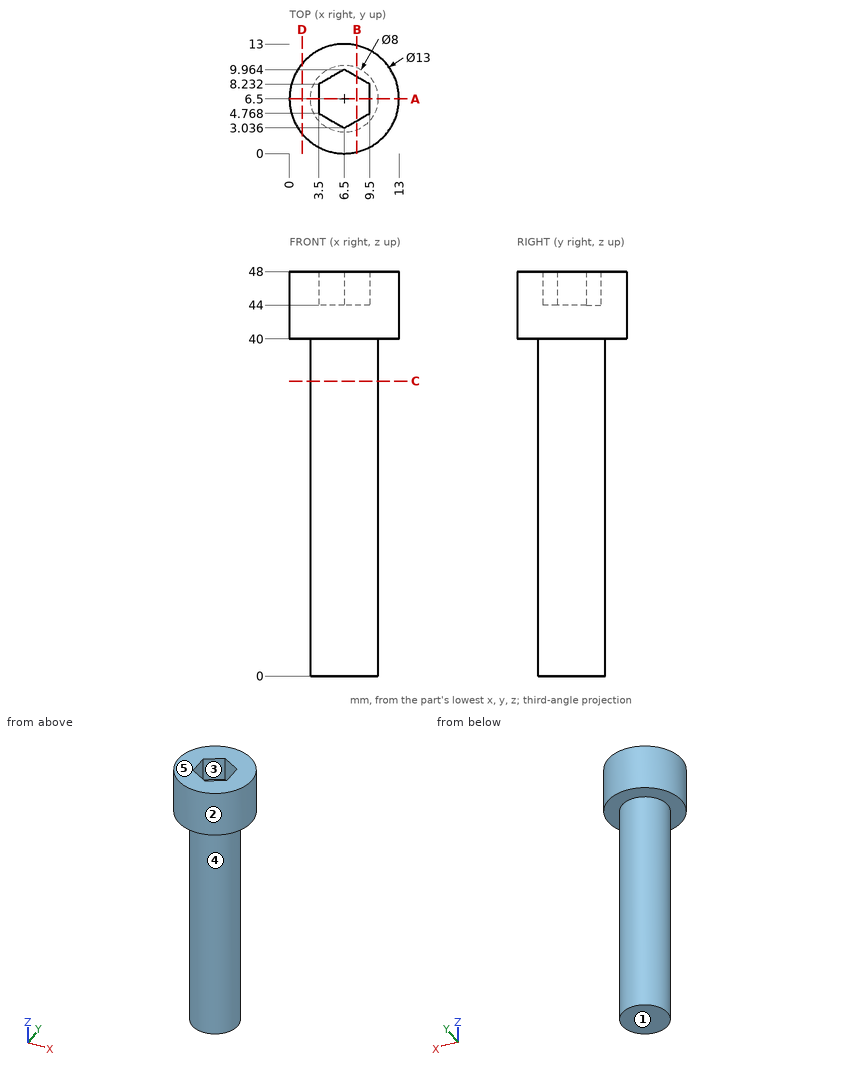
Source: three-view drawing plus pictorial views. Frame: mm from the lowest corner of the part. A direction names the side the tool comes from. Coordinates: 2 decimals unless noted, no trailing zeros. Order: outer loops, then holes, each group sorted by start corner. A loop starts at its lowest first (then second) coordinate and runs counter-clockwise, first axis right, second up. Notation, with made-up numbers: M 7.5,23.25 L 56.5,23.25 A28 cw 56.5,43.25 Z; hole C 1,-16.75 d9. An arc over 180 degrees is marked long. Answer in a Markdown table with one row per item.
(1) Material intervals for line 1 (Z direction, x = 6.5, y = 5); line 2 (Z direction, x = 12, y = 7); line 3 (Y direction, x = 6.25, z = 34), sorted ascending. Write a range as [from, to].
Numbers:
| item | result |
|---|---|
| line 1 | z = [0, 44] |
| line 2 | z = [40, 48] |
| line 3 | y = [2.51, 10.49] |
(2) Section query D-D, the plane x = 1.5. Output: boundary loops of the cut face in (y, z).
Numbers:
| item | result |
|---|---|
| outline | M 2.35,40 L 10.65,40 L 10.65,48 L 2.35,48 Z |
(3) Draft query along Y for the marked faces 1, 2 and 3. Return one class per face: pulls with the +Y half, pulls with the -Y half, needs draft (parallel to the pull), parting line crosses it, or undercut.
Numbers:
| item | result |
|---|---|
| face 1 | needs draft |
| face 2 | parting line crosses it |
| face 3 | undercut |
(4) Access query for the marked faces 4 and 5. Directions: +Z, -Z, +X, -X, +Y, -Y. A direction counts if a zero-diameter tool reaches every point of the face in a straight line with its end or side. Return the directions, or none.
Numbers:
| item | result |
|---|---|
| face 4 | -Z |
| face 5 | +Z, +X, -X, +Y, -Y |
(5) Section query C-C, the plane z = 35. Output: boundary loops of the cut face in (x, y).
Numbers:
| item | result |
|---|---|
| outline | C 6.5,6.5 d8 |
(6) Contact query for flat-ended pins moving along their axis: pin 1 Ø1.5 at (x, y) = (10.5, 6.5) entering from -Z; pin 2 Ø3 at (x, z) = (11, 20.5) entering from +Y; pin 3 Ø5 at (y, z) = (3, 20) entering from -X; pin 4 Ø3 at (y, z) = (1.5, 19) entering from -X. Output: stop coordinate, or through.
Numbers:
| item | result |
|---|---|
| pin 1 | stops at z = 0 |
| pin 2 | stops at y = 9.15 |
| pin 3 | stops at x = 2.63 |
| pin 4 | stops at x = 4.56 |
(7) Section query A-A, the plane y = 6.5. Output: boundary loops of the cut face in (x, z), plus the area to 3 significant figures.
Numbers:
| item | result |
|---|---|
| outline | M 0,40 L 2.5,40 L 2.5,0 L 10.5,0 L 10.5,40 L 13,40 L 13,48 L 9.5,48 L 9.5,44 L 3.5,44 L 3.5,48 L 0,48 Z |
| area | 400 mm^2 |
(8) Section query B-B, the plane x = 8. Output: boundary loops of the cut face in (y, z).
Numbers:
| item | result |
|---|---|
| outline | M 0.18,40 L 2.79,40 L 2.79,0 L 10.21,0 L 10.21,40 L 12.82,40 L 12.82,48 L 9.1,48 L 9.1,44 L 3.9,44 L 3.9,48 L 0.18,48 Z |
